Design review of the part shown in the three views and the two pictorial views. Dimensions are in mm from the part's minimum x, y and z. A direction names the side the tool comes from. Give positions to 0.01 mm unless a question says otherwise; leave off trailing zeros. Write each loop counter-clockwise with the first axis right and the second up, starting at its lowest first coordinate (ties: lowest second). Pieces come first, ordered by that corner, then holes. Notation, with made-up numbers: (-19.5, 0.5) -> (19.5, 0.5) arc R12 cw to (19.5, 23.5) -> close; hole circle Ø7 at (-4.75, -32). An arc over 180 degrees is marked (long way). Return JSON: item names as keys, results as strings. Group by question number.
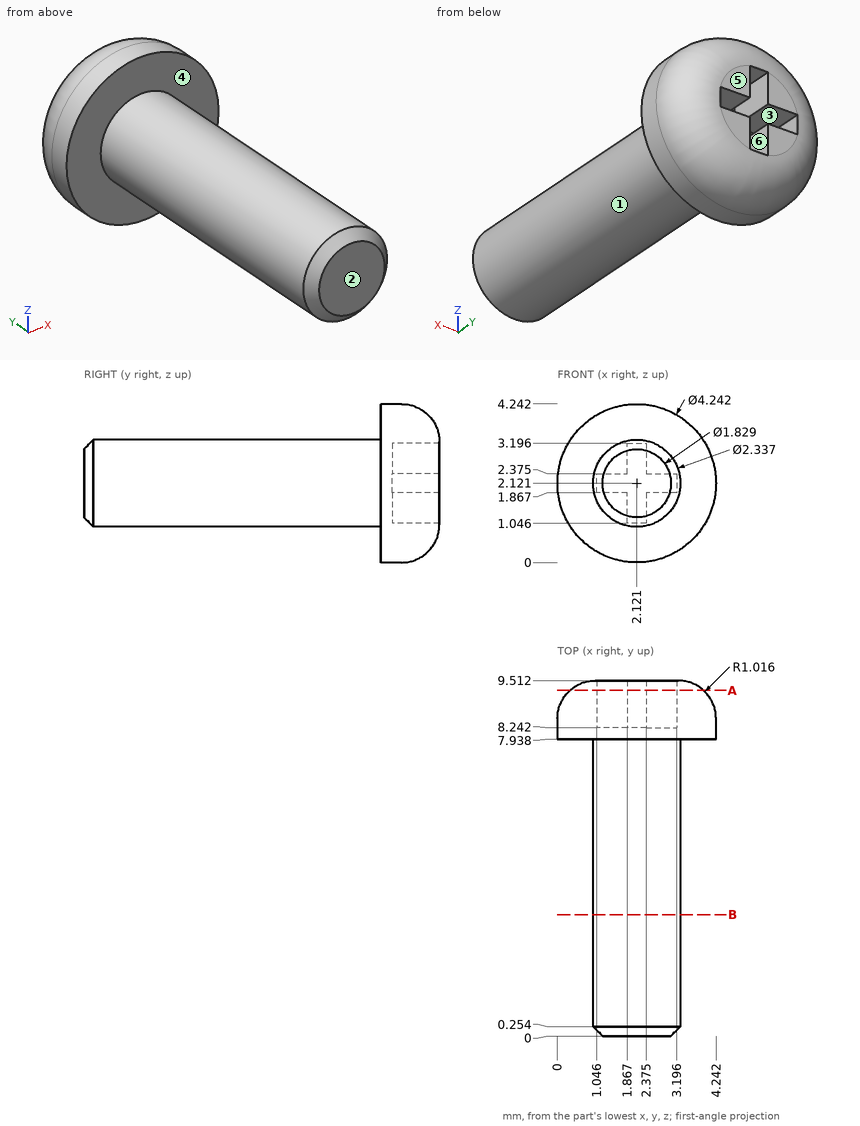
Q1. Tool access review of the marked faces 4, 5 and 6: name each direction out of +Z, -Z, +X, -X, +Y, -Y from which nothing blocks a thin tool from reaching the whole face with its end or side.
Q2. Take a section at A-A, the plane y = 9.25. Give the boundary of the cut face in (x, z) (1 decimal).
Q3. Insertion check: pin 1 (1.1 mm diameter, centred on x = 2.5, z = 2, fed in from +Y); pin 2 (0.6 mm diameter, centred on x = 2, y = 9, fed in from +Z); pin 3 (0.6 mm diameter, centred on y = 9, z = 2, fed in from -X); pin 4 (2 mm diameter, centred on y = 1.5, z = 1.5, fed in from +X). Each pin has a flat end and moves straight along its axis. Give the tip position at first contact, or say it passes through.
Q4. Mouldability with a two-part tool opening along Z and no side actions: class the marked faces 1, 2 and 3 as +Z half, -Z half, draft (parallel to the pull), parting line (faces both ways), or undercut.
Q5. Take a section at B-B, the plane y = 3.25. Give the boundary of the cut face in (x, z).
Q6. For L1, parallel to X at y = 4, z = 2.1; L2, parallel to X at y = 1, z = 1.75; L3, parallel to X at y = 9.25, z = 1.8 (1 decimal), list the stretches that pass through material, from the lowest coordinate up. Write a range as from..to.
Final values:
{
 "1": {"face 4": "-Y", "face 5": "+Z, -Z, +X, -X, +Y", "face 6": "+Y"},
 "2": {"outline": "circle Ø3.6 at (2.1, 2.1); hole (1, 1.9) -> (1.9, 1.9) -> (1.9, 1) -> (2.4, 1) -> (2.4, 1.9) -> (3.2, 1.9) -> (3.2, 2.4) -> (2.4, 2.4) -> (2.4, 3.2) -> (1.9, 3.2) -> (1.9, 2.4) -> (1, 2.4) -> close"},
 "3": {"pin 1": "stops at y = 9.51", "pin 2": "stops at z = 4.22", "pin 3": "stops at x = 0.02", "pin 4": "stops at x = 3.29"},
 "4": {"face 1": "parting line", "face 2": "draft", "face 3": "undercut"},
 "5": {"outline": "circle Ø2.34 at (2.12, 2.12)"},
 "6": {"L1": "x = 0.95..3.29", "L2": "x = 1.01..3.23", "L3": "x = 0.4..1.9, 2.4..3.9"}
}
